Read the model definition and answer for the solid it produces. Units are mm, in the model's axes. A direction names the side the tool comes from. Coordinates: 2 decimals unless noted, no trailing zeros. Order: outer loops, then holes, each group sorted by start corner. A loop starts at its lowest first (then second) coordinate and runs counter-clockwise, first axis right, second up. Notation, with made-up numbers: M 4,-21.5 L 18,-21.5 A16 ccw 18,-10.5 Z; hole C -31,62 d9. An arc over 180 degrees is marked long. Use a Markdown table: item, result. Add a question column.
1) Find the intervals of material crossed by probe 1 along Y at (x, z) = (0, 1.4) (3 decimals); probe 2 along Z at (x, y) = (-0.75, -2.25); probe 3 along Z at (x, y) = (3.75, -2.25), in increasing order. Write a range as [from, to].
2) For faces 4 (the face through (-0.3, -1.34, 5.73)), 5 (the face through (2.98, 0.94, 2.22)), 6 (the face through (-1.4, 3.1, 0)), determine the directions among +Z, -Z, +X, -X, +Y, -Y from which every point of the face is accessible in a straight line to the end or side of a thin tool.
3) Find section A-A on z = 4.25. Write down the section's boundary in (x, y) (3 decimals).
4) Find section B-B on x = 0. Write down the section's boundary in (y, z) (3 decimals).
5) Each of these flat-tipped pins is pushed along its axis until it touches: pin 1 Ø5 at (x, y) = (0, 0) entering from -Z; pin 2 Ø3 at (x, y) = (-3, 3) entering from -Z; pin 3 Ø4 at (x, y) = (-3.5, 5) entering from -Z. Where does it stop, or does it pass through?
6) Find section D-D on z = 2.75. Write down the section's boundary in (x, y) (3 decimals).
7) The mould has two halves that part along X. Classify faces 1 (the face through (0, -6, 3)), 2 (the face through (0.08, 7.25, -1.79)), 3 (the face through (-0.74, -1.35, 4.5)): released by +X, released by -X, zero draft, split by the parting line, or undercut.
8) Find section C-C on y = 1. Write down the section's boundary in (x, z).
from build123d import *

# Parameters (mm, degrees)
SKETCH114_R          = 1.375
PAD047_DEPTH         = 7
POCKET060_DEPTH      = 100
POCKET060_DEPTH_BACK = 100
SKETCH116_R          = 3.125
POCKET061_DEPTH      = 4.5
SKETCH117_W          = 12
SKETCH117_H          = 7.5
PAD048_DEPTH         = 2.5
FILLET025_R          = 2.49


with BuildPart() as part:
    # Sketch114 → Pad047 (new body)
    with BuildSketch(Plane.XY):
        with BuildLine():
            ThreePointArc((-6, 0), (0, -6), (6, 0))
            Line((6, 0), (6, 14))
            Line((-6, 14), (6, 14))
            Line((-6, 0), (-6, 14))
        make_face()
        Circle(SKETCH114_R, mode=Mode.SUBTRACT)
    extrude(amount=PAD047_DEPTH)

    # Sketch115 → Pocket060 (cut, two sides)
    with BuildSketch(Plane.YZ) as pocket060_sk:
        Polygon((0, 7), (14, 2), (14, 15.229534), align=None)
    extrude(amount=-POCKET060_DEPTH, mode=Mode.SUBTRACT)
    extrude(pocket060_sk.sketch, amount=POCKET060_DEPTH_BACK, mode=Mode.SUBTRACT)

    # Sketch116 → Pocket061 (cut)
    with BuildSketch(Plane.XY):
        Circle(SKETCH116_R)
    extrude(amount=POCKET061_DEPTH, mode=Mode.SUBTRACT)

    # Sketch117 → Pad048 (join)
    with BuildSketch(Plane.XY):
        with Locations((0, 10.25)):
            Rectangle(SKETCH117_W, SKETCH117_H)
    extrude(amount=-PAD048_DEPTH)

    # Fillet025
    fillet025_edges = [part.edges().sort_by_distance(p)[0] for p in [
        (0, 6.5, -2.5),
    ]]
    fillet(fillet025_edges, radius=FILLET025_R)


solid = part.part
Check result:
| question | item | result |
|---|---|---|
| 1 | probe 1 | y = [-6, -3.125], [3.125, 14] |
| 1 | probe 2 | z = [4.5, 7] |
| 1 | probe 3 | z = [0, 7] |
| 2 | face 4 | +Z, -Z |
| 2 | face 5 | -Z |
| 2 | face 6 | -Z, +X, -X, -Y |
| 3 | outline | M -6,0 A6 ccw 6,0 L 6,7.7 L -6,7.7 Z; hole C 0,0 d6.25 |
| 4 | outline | M -6,0 L -3.125,0 L -3.125,4.5 L -1.375,4.5 L -1.375,7 L -6,7 Z; M 1.375,4.5 L 3.125,4.5 L 3.125,0 L 6.5,0 L 6.5,-0.01 A2.49 ccw 8.99,-2.5 L 14,-2.5 L 14,2 L 1.375,6.509 Z |
| 5 | pin 1 | stops at z = 4.5 |
| 5 | pin 2 | stops at z = 0 |
| 5 | pin 3 | stops at z = -1.51 |
| 6 | outline | M -6,0 A6 ccw 6,0 L 6,11.9 L -6,11.9 Z; hole C 0,0 d6.25 |
| 7 | face 1 | split by the parting line |
| 7 | face 2 | zero draft |
| 7 | face 3 | undercut |
| 8 | outline | M -6,0 L -2.96,0 L -2.96,4.5 L -0.94,4.5 L -0.94,6.64 L -6,6.64 Z; M 0.94,4.5 L 2.96,4.5 L 2.96,0 L 6,0 L 6,6.64 L 0.94,6.64 Z |
